Verification items for this drawing (mm, ordinates from the low corner). A direction names the side the tool comes from. Give positions to 0.01 mm unless a question says otherwise; leave off trailing zeros. Loops run counter-clockwise (first coordinate to the right, second up) from the corner with the lowest first, then second, coordinate; pieces in that order, holes last. Notation, with made-up numbers: M 80,4 L 108,4 A14 ccw 108,10 Z; hole C 26.25,39.25 d5. An arc over 180 degrees is marked long. Put each result on its own line as item: value. Start each with the question number.
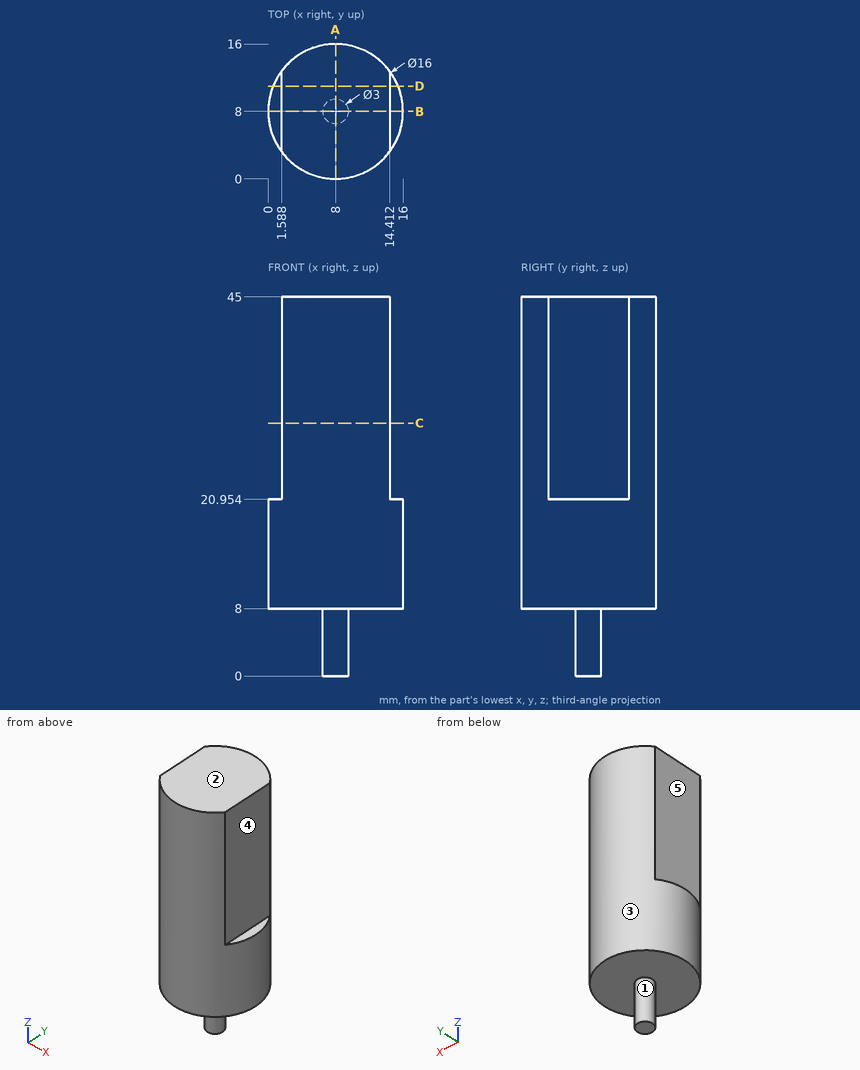
Q1. Set-up check for the marked faces 1, 2, 3, 4 and 5: record each of +Z, -Z, +X, -X, +Y, -Y from which the full face is reachable in a straight line by a thin tool's end or side.
Q2. Cross-section at A-A, the plane x = 8. Record the boundary of the cut face in (y, z), then the cut area to 3 significant figures.
Q3. Scan lines: L1, parallel to X at y = 12.5, z = 26; L2, parallel to Z at x = 1.5, y = 3.75 (1 decimal); L3, parallel to Z at x = 2.5, y = 4.75. Record each from-to range of solid material in increasing order.
Q4. Cross-section at B-B, the plane y = 8. Record the boundary of the cut face in (x, z) (1 decimal), then the cut area to 3 significant figures.
Q5. Cross-section at D-D, the plane y = 11. Record the boundary of the cut face in (x, z) (1 decimal).
Q6. Cross-section at C-C, the plane z = 30. Record the boundary of the cut face in (x, y).
Q7. Go/stop test with flat-tipped pins: pin 1 (6 mm diameter, centred on x = 2, z = 6, fed in from +Y); pin 2 (4 mm diameter, centred on y = 6.5, z = 28.5, fed in from +X); pin 3 (0.5 mm diameter, centred on x = 1, y = 6, fed in from +Z). Record where each tip stops, or that it passes through.
Ans:
1. face 1: -Z
1. face 2: +Z, +X, -X, +Y, -Y
1. face 3: +Z, -Z
1. face 4: +Z, +X, +Y, -Y
1. face 5: +Z, -X, +Y, -Y
2. outline: M 0,8 L 6.5,8 L 6.5,0 L 9.5,0 L 9.5,8 L 16,8 L 16,45 L 0,45 Z
2. area: 616 mm^2
3. L1: x = 1.59 to 14.41
3. L2: z = 8 to 21
3. L3: z = 8 to 45
4. outline: M 0,8 L 6.5,8 L 6.5,0 L 9.5,0 L 9.5,8 L 16,8 L 16,21 L 14.4,21 L 14.4,45 L 1.6,45 L 1.6,21 L 0,21 Z
4. area: 540 mm^2
5. outline: M 0.6,8 L 15.4,8 L 15.4,21 L 14.4,21 L 14.4,45 L 1.6,45 L 1.6,21 L 0.6,21 Z
6. outline: M 1.59,3.22 A8 ccw 14.41,3.22 L 14.41,12.78 A8 ccw 1.59,12.78 Z
7. pin 1: stops at y = 15.06
7. pin 2: stops at x = 14.41
7. pin 3: stops at z = 20.95
